Design review of the part built by this model. Coordinates are the model's own, in mm. A direction names the side the tool comes from. Round coordinates to 2 decimals unless told otherwise and drop trailing zeros. Write each loop counter-clockwise with the first axis right and the second up, starting at its lowest first coordinate (ties: lowest second). Pieces come first, ordered by that corner, then holes. Notation, with made-up numbers: M 38,44 L 58,44 A28 cw 58,62 Z; hole C 20,13.5 d3. An arc over 180 degrees is marked long. Use CSV: the item, a comma, the result in double quotes.
from build123d import *

# Parameters (mm, degrees)
EXTRUDE_1_DEPTH          = 20
SKETCH_2_W               = 6
SKETCH_2_H               = 10
CUT_EXTRUDE_1_DEPTH      = 20
EXTRUDE_2_DEPTH          = 5
EXTRUDE_2_DEPTH_BACK     = 5
SKETCH_3_W               = 8
SKETCH_3_H               = 20
EXTRUDE_3_DEPTH          = 5
EXTRUDE_3_DEPTH_BACK     = 5
SKETCH_4_W               = 20
SKETCH_4_H               = 20
CUT_EXTRUDE_2_DEPTH      = 52.23475383
CUT_EXTRUDE_2_DEPTH_BACK = 52.23475383
SKETCH_5_W               = 80.386179801
SKETCH_5_H               = 26.605581219
SKETCH_6_R               = 2
CUT_EXTRUDE_3_DEPTH      = 49.989794856
CHAMFER_1_SIZE           = 0.5
FILLET_1_R               = 10
SKETCH_7_W               = 5
SKETCH_7_H               = 20
EXTRUDE_4_DEPTH          = 10
SKETCH_8_R               = 64.5
EXTRUDE_5_DEPTH          = 4
SKETCH_9_W               = 60
SKETCH_9_H               = 60
SKETCH_9_W_2             = 85.907763787
SKETCH_9_H_2             = 140
CUT_EXTRUDE_4_DEPTH      = 5
EXTRUDE_8_DEPTH          = 37
EXTRUDE_9_DEPTH          = 4
SKETCH_15_W              = 8
SKETCH_15_H              = 10
EXTRUDE_10_DEPTH         = 3
SKETCH_16_R              = 2
CUT_EXTRUDE_5_DEPTH      = 3
FILLET_START             = -51.5
FILLET_2_DEPTH           = 2.999999733
FILLET_START_2           = 61.5
FILLET_2_2_DEPTH         = 2.999999733
FILLET_START_3           = -44.499993891
FILLET_2_3_DEPTH         = 2.999993891
FILLET_START_4           = 68.500006109
FILLET_2_4_DEPTH         = 2.999993891
FILLET_START_5           = -48.500000267
FILLET_2_5_DEPTH         = 4.000006376
FILLET_START_6           = 64.499999733
FILLET_2_6_DEPTH         = 4.000006376
FILLET_START_7           = 3
FILLET_2_7_OUTLINE_R     = 2
FILLET_2_7_DEPTH         = 3.797947653


with BuildPart() as part:
    # 草图1 → 凸台-拉伸1 (new body)
    with BuildSketch(Plane(origin=(0, 0, 0), x_dir=(1, 0, 0), z_dir=(0, 1, 0))):
        with BuildLine():
            Line((32, 17.82359333), (32, -17.82359333))
            Line((32, -17.82359333), (6.015712619, -24.265432238))
            ThreePointArc((6.015712619, -24.265432238), (-25, 0), (6.015712619, 24.265432238))
            Line((6.015712619, 24.265432238), (32, 17.82359333))
        make_face()
        with BuildLine():
            Line((22, 10), (22, -10))
            Line((22, -10), (3.609427572, -14.559259343))
            ThreePointArc((3.609427572, -14.559259343), (-15, 0), (3.609427572, 14.559259343))
            Line((3.609427572, 14.559259343), (22, 10))
        make_face(mode=Mode.SUBTRACT)
    extrude(amount=EXTRUDE_1_DEPTH)

    # 草图2 → 切除-拉伸1 (cut)
    with BuildSketch(Plane(origin=(0, 20, 0), x_dir=(1, 0, 0), z_dir=(0, 1, 0))):
        with Locations((25, 0)):
            Rectangle(SKETCH_2_W, SKETCH_2_H)
    extrude(amount=-CUT_EXTRUDE_1_DEPTH, mode=Mode.SUBTRACT)

    # 草图3 → 凸台-拉伸2 (add, two sides: drawn at the far end of the back side and taken through both)
    with BuildSketch(Plane.XY.offset(-EXTRUDE_2_DEPTH_BACK)):
        with Locations((36, 10)):
            Rectangle(SKETCH_3_W, SKETCH_3_H)
    extrude(amount=EXTRUDE_2_DEPTH + EXTRUDE_2_DEPTH_BACK)

    # 草图4 → 凸台-拉伸3 (add, two sides: drawn at the far end of the back side and taken through both)
    with BuildSketch(Plane.XY.offset(-EXTRUDE_3_DEPTH_BACK)):
        with Locations((-25, 10)):
            Rectangle(SKETCH_4_W, SKETCH_4_H)
    extrude(amount=EXTRUDE_3_DEPTH + EXTRUDE_3_DEPTH_BACK)

    # 草图5 → 切除-拉伸2 (cut, two sides: drawn at the far end of the back side and taken through both)
    with BuildSketch(Plane(origin=(0, 20, 0), x_dir=(1, 0, 0), z_dir=(0, 1, 0)).offset(-CUT_EXTRUDE_2_DEPTH_BACK)):
        with Locations((-0.193089901, 13.30279061)):
            Rectangle(SKETCH_5_W, SKETCH_5_H)
    extrude(amount=CUT_EXTRUDE_2_DEPTH + CUT_EXTRUDE_2_DEPTH_BACK, mode=Mode.SUBTRACT)

    # 草图6 → 切除-拉伸3 (cut, through all)
    with BuildSketch(Plane.XY.offset(5)):
        with Locations((-30, 10)):
            Circle(SKETCH_6_R)
        with Locations((36, 10)):
            Circle(SKETCH_6_R)
    extrude(amount=-CUT_EXTRUDE_3_DEPTH, mode=Mode.SUBTRACT)

    # 倒角1
    chamfer_1_edges = [part.edges().sort_by_distance(p)[0] for p in [
        (-32, 10, 5),
        (34, 10, 5),
    ]]
    chamfer(chamfer_1_edges, length=CHAMFER_1_SIZE)

    # 圆角1
    fillet_1_edges = [part.edges().sort_by_distance(p)[0] for p in [
        (32, 10, 17.82359333),
    ]]
    fillet(fillet_1_edges, radius=FILLET_1_R)

    # 草图7 → 凸台-拉伸4 (add)
    with BuildSketch(Plane.ZY.offset(35)):
        with Locations((2.5, 10)):
            Rectangle(SKETCH_7_W, SKETCH_7_H)
    extrude(amount=EXTRUDE_4_DEPTH)

    # 草图8 → 凸台-拉伸5 (add)
    with BuildSketch(Plane.ZY.offset(45)):
        with Locations((0, 10)):
            Circle(SKETCH_8_R)
    extrude(amount=EXTRUDE_5_DEPTH)

    # 草图9 → 切除-拉伸4 (cut)
    with BuildSketch(Plane(origin=(-45, 0, 0), x_dir=(0, 0, -1), z_dir=(1, 0, 0))):
        with Locations((-45, 50)):
            Rectangle(SKETCH_9_W, SKETCH_9_H)
        with Locations((-45, -30)):
            Rectangle(SKETCH_9_W, SKETCH_9_H)
        with Locations((42.953881894, 10)):
            Rectangle(SKETCH_9_W_2, SKETCH_9_H_2)
    extrude(amount=-CUT_EXTRUDE_4_DEPTH, mode=Mode.SUBTRACT)

    # 草图11 → 凸台-拉伸8 (add)
    with BuildSketch(Plane.ZY.offset(49)):
        with BuildLine():
            ThreePointArc((60.681545794, 20), (61.5, 10), (60.681545794, 0))
            Line((60.681545794, 0), (63.720091023, 0))
            ThreePointArc((63.720091023, 0), (64.5, 10), (63.720091023, 20))
            Line((63.720091023, 20), (60.681545794, 20))
        make_face()
        with BuildLine():
            Line((0, 74.5), (0, 71.5))
            ThreePointArc((0, 71.5), (7.557274891, 71.0339053), (15, 69.642686056))
            Line((15, 69.642686056), (15, 72.731570999))
            ThreePointArc((15, 72.731570999), (7.551942484, 74.05636709), (0, 74.5))
        make_face()
        with BuildLine():
            ThreePointArc((15, -49.642686056), (7.557274891, -51.0339053), (0, -51.5))
            Line((0, -51.5), (0, -54.5))
            ThreePointArc((0, -54.5), (7.551942484, -54.05636709), (15, -52.731570999))
            Line((15, -52.731570999), (15, -49.642686056))
        make_face()
    extrude(amount=EXTRUDE_8_DEPTH)

    # 草图13 → 凸台-拉伸9 (add)
    with BuildSketch(Plane.ZY.offset(86)):
        with BuildLine():
            Line((63.720091023, 20), (38.720091023, 20))
            Line((38.720091023, 20), (38.720091023, 0))
            Line((38.720091023, 0), (63.720091023, 0))
            ThreePointArc((63.720091023, 0), (64.5, 10), (63.720091023, 20))
        make_face()
        with BuildLine():
            Line((0, -54.5), (0, -27.731570999))
            Line((0, -27.731570999), (15, -27.731570999))
            Line((15, -27.731570999), (15, -52.731570999))
            ThreePointArc((15, -52.731570999), (7.551942484, -54.05636709), (0, -54.5))
        make_face()
        with BuildLine():
            Line((0, 74.5), (0, 49.5))
            Line((0, 49.5), (15, 49.5))
            Line((15, 49.5), (15, 72.731570999))
            ThreePointArc((15, 72.731570999), (7.551942484, 74.05636709), (0, 74.5))
        make_face()
    extrude(amount=EXTRUDE_9_DEPTH)

    # 草图15 → 凸台-拉伸10 (add)
    with BuildSketch(Plane(origin=(0, 0, 0), x_dir=(-1, 0, 0), z_dir=(0, 0, -1))):
        with Locations((94, 66.5)):
            Rectangle(SKETCH_15_W, SKETCH_15_H)
        with Locations((94, -46.5)):
            Rectangle(SKETCH_15_W, SKETCH_15_H)
    extrude(amount=-EXTRUDE_10_DEPTH)

    # 草图16 → 切除-拉伸5 (cut)
    with BuildSketch(Plane.XY.offset(3)):
        with Locations((-94, 66.5)):
            Circle(SKETCH_16_R)
        with Locations((-94, -46.5)):
            Circle(SKETCH_16_R)
    extrude(amount=-CUT_EXTRUDE_5_DEPTH, mode=Mode.SUBTRACT)

    # 圆角2: read off the stored shape, not the designer's step
    # 圆角2 outline → 圆角2 (add)
    with BuildSketch(Plane(origin=(0, 0, 0), x_dir=(1, 0, 0), z_dir=(0, 1, 0)).offset(FILLET_START)):
        with BuildLine():
            ThreePointArc((-98, -3), (-92.254033308, -6.473403651), (-90, -12.797958971))
            Line((-90, -12.797958971), (-90, -3))
            Line((-90, -3), (-98, -3))
        make_face()
    extrude(amount=FILLET_2_DEPTH)

    # Fillet 2 2 outline → Fillet 2 2 (add)
    with BuildSketch(Plane(origin=(0, 0, 0), x_dir=(1, 0, 0), z_dir=(0, 1, 0)).offset(FILLET_START_2)):
        with BuildLine():
            ThreePointArc((-98, -3), (-92.254033308, -6.473403651), (-90, -12.797958971))
            Line((-90, -12.797958971), (-90, -3))
            Line((-90, -3), (-98, -3))
        make_face()
    extrude(amount=FILLET_2_2_DEPTH)

    # Fillet 2 3 outline → Fillet 2 3 (add)
    with BuildSketch(Plane(origin=(0, 0, 0), x_dir=(1, 0, 0), z_dir=(0, 1, 0)).offset(FILLET_START_3)):
        with BuildLine():
            ThreePointArc((-98, -3), (-92.254033308, -6.473403651), (-90, -12.797958971))
            Line((-90, -12.797958971), (-90, -3))
            Line((-90, -3), (-98, -3))
        make_face()
    extrude(amount=FILLET_2_3_DEPTH)

    # Fillet 2 4 outline → Fillet 2 4 (add)
    with BuildSketch(Plane(origin=(0, 0, 0), x_dir=(1, 0, 0), z_dir=(0, 1, 0)).offset(FILLET_START_4)):
        with BuildLine():
            ThreePointArc((-98, -3), (-92.254033308, -6.473403651), (-90, -12.797958971))
            Line((-90, -12.797958971), (-90, -3))
            Line((-90, -3), (-98, -3))
        make_face()
    extrude(amount=FILLET_2_4_DEPTH)

    # Fillet 2 5 outline → Fillet 2 5 (add)
    with BuildSketch(Plane(origin=(0, 0, 0), x_dir=(1, 0, 0), z_dir=(0, 1, 0)).offset(FILLET_START_5)):
        with BuildLine():
            ThreePointArc((-98, -3), (-92.254033308, -6.473403651), (-90, -12.797958971))
            Line((-90, -12.797958971), (-90, -3))
            Line((-90, -3), (-98, -3))
        make_face()
    extrude(amount=FILLET_2_5_DEPTH)

    # Fillet 2 6 outline → Fillet 2 6 (add)
    with BuildSketch(Plane(origin=(0, 0, 0), x_dir=(1, 0, 0), z_dir=(0, 1, 0)).offset(FILLET_START_6)):
        with BuildLine():
            ThreePointArc((-98, -3), (-92.254033308, -6.473403651), (-90, -12.797958971))
            Line((-90, -12.797958971), (-90, -3))
            Line((-90, -3), (-98, -3))
        make_face()
    extrude(amount=FILLET_2_6_DEPTH)

    # Fillet 2 7 outline → Fillet 2 7 (cut)
    with BuildSketch(Plane.XY.offset(FILLET_START_7)):
        with Locations((-94, 66.5)):
            Circle(FILLET_2_7_OUTLINE_R)
        with Locations((-94, -46.5)):
            Circle(FILLET_2_7_OUTLINE_R)
    extrude(amount=FILLET_2_7_DEPTH, mode=Mode.SUBTRACT)


solid = part.part
1) The part is to be moulded in two halves that separate along X. For faces 1 (the face through (-86, 10, 50)), 2 (the face through (-86, 61, 7)), 3 (the face through (-62, -50, 15)), 4 (the face through (-91.434, 66.43, 7.638)), say which applies: released by +X, released by -X, zero draft, split by the parting line, or undercut.
Answers:
face 1,"undercut"
face 2,"undercut"
face 3,"zero draft"
face 4,"released by -X"
2) Add section A-A on z = 55. Write out the cut boundary in (x, y), then the cut area to 3 significant figures.
Answers:
outline,"M -90,0 L -86,0 L -86,20 L -90,20 Z; M -49,0 L -45,0 L -45,20 L -49,20 Z"
area,"160 mm²"
3) Add section D-D on x = -94. Write out the cut boundary in (y, z).
Answers:
outline,"M -51.5,0 L -48.5,0 L -48.5,4.8 L -51.5,4.8 Z; M -44.5,0 L -41.5,0 L -41.5,4.8 L -44.5,4.8 Z; M 61.5,0 L 64.5,0 L 64.5,4.8 L 61.5,4.8 Z; M 68.5,0 L 71.5,0 L 71.5,4.8 L 68.5,4.8 Z"
4) Machinability: for faces 5 (the face through (32, 10, 7)), 6 (the face through (-67.2, 10.1, 61.5)), 7 (the face through (-93, -51.5, 3)), 8 (the face through (-64, 0, 61)), 9 (the face through (-64, 70, 15)), which of the approach directions +Z, -Z, +X, -X, +Y, -Y give a long, thin tool a straight path to every point of the face, cutting with its end or side? Answer none if there is none.
Answers:
face 5,"+Z, +X, +Y, -Y"
face 6,"-Z"
face 7,"+Z, -Z, -X, -Y"
face 8,"+Z, +X, -X, -Y"
face 9,"+Z, +X, -X, +Y"
5) For pin 1 Ø5 at (x, y) = (26, 2.5) entering from +Z; pin 2 Ø4.5 at (x, z) = (-89, 9) entering from +Y; pin 3 Ø12 at (y, z) = (-7.5, 48.5) entering from +X; pin 4 Ø8 at (y, z) = (6.5, 48.5) entering from -X, all flat-tipped, find the tip position at first contact; note any pin that passes through.
Answers:
pin 1,"z = 19.93"
pin 2,"y = 74.15"
pin 3,"through"
pin 4,"x = -90"
6) Add section C-C on x = 36. Write out the cut boundary in (y, z).
Answers:
outline,"M 0,0 L 8,0 L 8,4.5 L 7.5,5 L 0,5 Z; M 12,0 L 20,0 L 20,5 L 12.5,5 L 12,4.5 Z"
7) Add section B-B on y = 10. Give the number of separate pieces and of enclosed holes in the cut face, then the cut area to 3 significant figures.
Answers:
separate pieces,"3"
enclosed holes,"0"
area,"1,260 mm²"
8) Wall thickness on line 1 along Y through (x, z) = (-94, 1.75); line 2 along Y through (x, z) = (-30, 2); line 3 along X through (y, z) = (-46.5, 4.25): over which ranges is each line inside the solid? List them lowest first. Write a range as [from, to].
Answers:
line 1,"[-51.5, -48.5], [-44.5, -41.5], [61.5, 64.5], [68.5, 71.5]"
line 2,"[0, 8], [12, 20]"
line 3,"[-92, -86], [-49, -45]"
